```python
from build123d import *

# Parameters (mm, degrees)
SKETCH1_W          = 424
SKETCH1_H          = 103
BASE_FLANGE1_DEPTH = 4
SKETCH4_W          = 4
SKETCH4_H          = 20
TAB1_DEPTH         = 4
CUT_EXTRUDE1_DEPTH = 223.090634652


# Sheet-metal steps are written as plain solids
with BuildPart() as part:
    # Sketch1 → Base-Flange1 (new body)
    with BuildSketch(Plane.XY):
        Rectangle(SKETCH1_W, SKETCH1_H)
    extrude(amount=-BASE_FLANGE1_DEPTH)

    # Sketch4 → Tab1 (add)
    with BuildSketch(Plane.XY):
        with Locations((-214, 25)):
            Rectangle(SKETCH4_W, SKETCH4_H)
        with Locations((-214, -25)):
            Rectangle(SKETCH4_W, SKETCH4_H)
        with Locations((214, 25)):
            Rectangle(SKETCH4_W, SKETCH4_H)
        with Locations((214, -25)):
            Rectangle(SKETCH4_W, SKETCH4_H)
    extrude(amount=-TAB1_DEPTH)

    # Sketch5 → Cut-Extrude1 (cut, through all)
    with BuildSketch(Plane.XY):
        Polygon((-212, 1.75), (-209, 1.75), (-209, 2.75), (-205, 2.75), (-205, 1.75), (-200, 1.75), (-200, -1.75), (-205, -1.75), (-205, -2.75), (-209, -2.75), (-209, -1.75), (-212, -1.75), align=None)
        Polygon((212, -1.75), (212, 1.75), (209, 1.75), (209, 2.75), (205, 2.75), (205, 1.75), (200, 1.75), (200, -1.75), (205, -1.75), (205, -2.75), (209, -2.75), (209, -1.75), align=None)
    extrude(amount=-CUT_EXTRUDE1_DEPTH, mode=Mode.SUBTRACT)


solid = part.part
```
Here's how the part is built. I have some questions about the finished solid (model axes, mm). Give positions to 0.01 mm unless a question says otherwise; leave off trailing zeros. Order: outer loops, then holes, each group sorted by start corner. A loop starts at its lowest first (then second) coordinate and runs counter-clockwise, first axis right, second up. Notation, with made-up numbers: M 6,-37 L 25,-37 A24 cw 25,2 Z; hole C 7.5,-25.5 d4. An arc over 180 degrees is marked long. Use a Markdown table: item, result. Add a question column.
1. For pin 1 Ø1 at (y, z) = (0.5, -1.5) entering from -X; pin 2 Ø2 at (y, z) = (47, -2) entering from -X; pin 3 Ø4 at (x, y) = (132, 38.5) entering from +Z; pin 4 Ø1.2 at (x, z) = (-214.5, -3) entering from -Y, each with a flat end and sliding along its axis, tell me the tip position at first contact or that it passes through.
2. I need wall thicknesses on probe 1 along X at (y, z) = (7, -0.5); probe 2 along X at (y, z) = (1.5, -1.6). Which ranges of each line are inside material? Lowest first, please. Write a range as from..to.
3. Suppose I cut it at A-A (y = 39). List the corners of the cut face in (x, z) for me.
Results list:
| question | item | result |
|---|---|---|
| 1 | pin 1 | stops at x = -200 |
| 1 | pin 2 | stops at x = -212 |
| 1 | pin 3 | stops at z = 0 |
| 1 | pin 4 | stops at y = -35 |
| 2 | probe 1 | x = -212..212 |
| 2 | probe 2 | x = -200..200 |
| 3 | outline | M -212,-4 L 212,-4 L 212,0 L -212,0 Z |
